Autodesk Inventor part; units mm, degrees
ref_plane "YZ Plane" through (0, 0, 0) normal (1, 0, 0) x (0, 1, 0)
ref_plane "XZ Plane" through (0, 0, 0) normal (0, 1, 0) x (-1, 0, 0)
ref_plane "XY Plane" through (0, 0, 0) normal (0, 0, 1) x (1, 0, 0)
sketch "スケッチ1" plane through (0, 0, 0) normal (0, 0, 1) x (1, 0, 0)
  line L0 (0, 0) -> (20, 0)
  line L1 (20, 0) -> (20, 120)
  line L2 (20, 120) -> (0, 120)
  line L3 (0, 120) -> (0, 0)
  dimension "d0" = 120
  dimension "d1" = 20
extrude "押し出し1" add sketch "スケッチ1" along normal blind 2
sketch "スケッチ2" plane through (0, 0, 2) normal (0, 0, 1) x (1, 0, 0)
  line L0 (0, 0) -> (20, 0)
  line L1 (17.5, 0) -> (17.5, 120.1891) construction
  line L2 (20, 0) -> (20, 120)
  arc A0 (17.5, 19.55) -> (17.5, 9.45) centre (17.5, 14.5) ccw
  line L3 (17.5, 19.55) -> (20, 19.55)
  line L4 (17.5, 9.45) -> (20, 9.45)
  dimension "d4" = 2.5
  dimension "d5" = 14.5
  dimension "d6" = 10.1
extrude "押し出し2" cut sketch "スケッチ2" against normal up to surface (2 mm away)
sketch "スケッチ3" plane through (0, 0, 2) normal (0, 0, 1) x (1, 0, 0)
  arc A0 (17.5, 19.55) -> (17.5, 9.45) centre (17.5, 14.5) ccw
  circle A1 centre (17.5, 14.5) radius 8.5 construction
  point P0 (0, 0)
  point P1 (9, 14.5)
  point P2 (17.5, 23)
  point P3 (17.5, 6)
  dimension "d9" = 17
hole "穴1" at (9, 14.5, 2) at (17.5, 23, 2) at (17.5, 6, 2) direction (0, 0, -1) diameter 2.7 end through all
sketch "スケッチ4" plane through (0, 0, 2) normal (0, 0, 1) x (1, 0, 0)
  line L0 (20, 120) -> (0, 120)
  line L1 (4, 120) -> (4, 0) construction
  line L2 (0, 120) -> (0, 0)
  point P0 (4, 115.5)
  point P1 (4, 95.5)
  dimension "d17" = 4
  dimension "d18" = 4.5
  dimension "d19" = 20
hole "穴2" at (4, 115.5, 2) at (4, 95.5, 2) direction (0, 0, -1) diameter 2.4 end through all
sketch "スケッチ5" plane through (0, 0, 2) normal (0, 0, 1) x (1, 0, 0)
  line L0 (13, 111.275) -> (18, 111.275)
  line L1 (18, 111.275) -> (18, 101.275)
  line L2 (18, 101.275) -> (13, 101.275)
  line L3 (13, 101.275) -> (13, 111.275)
  line L4 (20, 19.55) -> (20, 120)
  circle A0 centre (18, 110.275) radius 1
  circle A1 centre (13, 110.275) radius 1
  circle A2 centre (13, 102.275) radius 1
  circle A3 centre (18, 102.275) radius 1
  point P0 (0, 0)
  dimension "d27" = 5
  dimension "d28" = 10
  dimension "d29" = 2
  dimension "d30" = 2
  dimension "d31" = 2
  dimension "d32" = 2
  dimension "d33" = 2
extrude "押し出し3" cut sketch "スケッチ5" against normal up to surface (2 mm away)
sketch "スケッチ6" plane through (0, 0, 2) normal (0, 0, 1) x (1, 0, 0)
  line L0 (15.5, 119.9651) -> (15.5, 0) construction
  line L1 (0, 0) -> (20, 0)
  line L2 (18, 109.275) -> (18, 103.275)
  line L3 (18, 106.275) -> (13, 106.275) construction
  line L4 (13, 103.275) -> (13, 109.275)
  point P0 (15.5, 116.275)
  point P1 (15.5, 96.275)
  dimension "d37" = 2.5
  dimension "d38" = 20
hole "穴3" at (15.5, 116.275, 2) at (15.5, 96.275, 2) direction (0, 0, -1) diameter 3.1 end through all
sketch "スケッチ7" plane through (0, 0, 2) normal (0, 0, 1) x (1, 0, 0)
  line L0 (20, 120) -> (0, 120)
  line L1 (10, 120) -> (10, 0) construction
  line L2 (0, 0) -> (20, 0)
  line L3 (8, 88.5) -> (12, 88.5)
  line L4 (14, 88.5) -> (14, 83.5)
  line L5 (12, 83.5) -> (8, 83.5)
  line L6 (6, 83.5) -> (6, 88.5)
  arc A0 (8, 88.5) -> (6, 88.5) centre (7, 88.5) ccw
  line L7 (6, 86) -> (14, 86) construction
  arc A1 (6, 83.5) -> (8, 83.5) centre (7, 83.5) ccw
  arc A2 (14, 88.5) -> (12, 88.5) centre (13, 88.5) ccw
  arc A3 (12, 83.5) -> (14, 83.5) centre (13, 83.5) ccw
  dimension "d48" = 8
  dimension "d49" = 5
  dimension "d50" = 2
  dimension "d64" = 34
extrude "押し出し5" cut sketch "スケッチ7" against normal through all
sketch "スケッチ9" plane through (0, 0, 2) normal (0, 0, 1) x (1, 0, 0)
  line L0 (0, 86) -> (19.9715, 86) construction
  line L1 (8, 88.5) -> (12, 88.5)
  line L2 (10, 88.5) -> (10, 71.9666) construction
  point P0 (0, 0)
  point P1 (2.5, 86)
  point P2 (17.5, 86)
  dimension "d55" = 2.5
  dimension "d56" = 15
hole "穴4" at (2.5, 86, 2) at (17.5, 86, 2) direction (0, 0, -1) diameter 3.1 end through all
fillet "フィレット3" radius 2 5 edges at (20, 0, 1) (20, 9.45, 1) (20, 19.55, 1) (20, 120, 1) (0, 120, 1)
fillet "フィレット4" radius 16 1 edges at (0, 0, 1)
thicken "厚み1" operation cut thickness 0.05 both sides no extend neighbours no toward (-1, 0, 0) faces at (6, 86.8333, 1.3333) (7.7994, 89.1007, 0.6667) (10.6667, 88.5, 0.6667) (12.1548, 89.0345, 0.6667) (6.2006, 82.8993, 0.6667) (9.3333, 83.5, 1.3333) (12.08, 83.108, 0.6667) (14, 85.1667, 1.3333)
thicken "厚み2" operation cut thickness 0.05 both sides no extend neighbours no toward (1, 0, 0) faces at (18, 107.275, 1.3333) (18.866, 110.775, 0.6667) (18.9035, 101.8464, 1.3333) (16.3333, 101.275, 1.3333) (12.0008, 102.2348, 0.6667) (13, 105.275, 1.3333) (12.134, 109.775, 0.6667) (14.6667, 111.275, 1.3333)
equation "\"d37\" = 0.5 * d27"
equation "\"d55\" = 0.5 * d49"
properties material "アルミニウム 2014-T4"
Can you work these out from the model? Positions are in its coordinate system, mm. A direction names the side the tool comes from. Give positions to 0.01 mm unless a question says otherwise; leave off trailing zeros. Loops run counter-clockwise (first coordinate to the right, second up) from the corner with the lowest first, then second, coordinate; pieces in that order, holes last. Notation, with made-up numbers: M 43.5,68.5 L 99.5,68.5 A19 ccw 99.5,73.5 Z; hole C 38,76 d11. An arc over 180 degrees is marked long. One line per item, written item: value.
(1) Which directions (+Z, -Z, +X, -X, +Y, -Y) give clear straight access to the entire face, cutting with the end or side of a thin tool? Please do faces 1 (the face through (19.43, 119.4, 1.01)), 2 (the face through (7, 89.55, 1.01)), 3 (the face through (19.4, 8.88, 0.99)).
Returned:
face 1: +Z, -Z, +X, +Y
face 2: +Z, -Z
face 3: +Z, -Z, +X
(2) We'd pull the mould along X, two halves only. Please class faces 4 (the face through (15, 111.325, 1)), 5 (the face through (20, 5, 1)), 6 (the face through (0, 68, 1)), 7 (the face through (17.094, 4.712, 0.986)): released by +X, released by -X, zero draft, split by the parting line, or undercut.
Returned:
face 4: undercut
face 5: released by +X
face 6: released by -X
face 7: undercut
(3) Suppose I cut it at A-A on y = 6. List the corners of the cut face in (x, z) for me, plus the area to 3 significant figures.
Returned:
outline: M 3.51,0 L 16.15,0 L 16.15,2 L 3.51,2 Z; M 18.85,0 L 20,0 L 20,2 L 18.85,2 Z
area: 27.6 mm^2
(4) Suppose I cut it at C-C on y = 23. List the corners of the cut face in (x, z) for me, plus the area to 3 significant figures.
Returned:
outline: M 0,0 L 16.15,0 L 16.15,2 L 0,2 Z; M 18.85,0 L 20,0 L 20,2 L 18.85,2 Z
area: 34.6 mm^2
(5) Will these pins go through, and if not, where does the flat tip stop? pin 1 (1.9 mm diameter, centred on x = 17.5, y = 86, fed in from -Z); pin 2 (1 mm diameter, centred on x = 14.5, z = 1, fed in from -Y).
Returned:
pin 1: through
pin 2: y = 0.03
(6) I need wall thicknesses on line 1 (X direction, y = 86, z = 1.05); line 2 (Y direction, x = 17.5, z = 0.6) (3 decimals); line 3 (X direction, y = 23, z = 0.6). Which ranges of each line are inside material? Lowest first, please.
Returned:
line 1: 0 to 0.95, 4.05 to 5.95, 14.05 to 15.95, 19.05 to 20
line 2: 0 to 4.65, 7.35 to 9.45, 19.55 to 21.65, 24.35 to 84.45, 87.55 to 101.225, 111.325 to 120
line 3: 0 to 16.15, 18.85 to 20
(7) Suppose I cut it at B-B on z = 1.65. Count the separate pieces of the cut face and the enclosed holes in it, plus the area to 3 significant figures.
Returned:
separate pieces: 1
enclosed holes: 11
area: 2,110 mm^2
